from build123d import *

# Parameters (mm, degrees)
ESQUISSE1_W             = 330
ESQUISSE1_H             = 238
BOSS_EXTRU_1_DEPTH      = 6
ESQUISSE2_W             = 20
ESQUISSE2_H             = 6
ESQUISSE2_W_2           = 30
BOSS_EXTRU_2_DEPTH      = 6
ESQUISSE3_W             = 6
ESQUISSE3_H             = 10
ENL_V_MAT_EXTRU_1_DEPTH = 6
ESQUISSE4_R             = 1.4
ENL_V_MAT_EXTRU_2_DEPTH = 6


with BuildPart() as part:
    # Esquisse1 → Boss.-Extru.1 (new body)
    with BuildSketch(Plane.XY):
        Rectangle(ESQUISSE1_W, ESQUISSE1_H)
    extrude(amount=BOSS_EXTRU_1_DEPTH)

    # Esquisse2 → Boss.-Extru.2 (add)
    with BuildSketch(Plane.XY.offset(6)):
        with Locations((-125, 122)):
            Rectangle(ESQUISSE2_W, ESQUISSE2_H)
        with Locations((-50, 122)):
            Rectangle(ESQUISSE2_W_2, ESQUISSE2_H)
        with Locations((50, 122)):
            Rectangle(ESQUISSE2_W_2, ESQUISSE2_H)
        with Locations((125, 122)):
            Rectangle(ESQUISSE2_W, ESQUISSE2_H)
        with Locations((125, -122)):
            Rectangle(ESQUISSE2_W, ESQUISSE2_H)
        with Locations((50, -122)):
            Rectangle(ESQUISSE2_W_2, ESQUISSE2_H)
        with Locations((-50, -122)):
            Rectangle(ESQUISSE2_W_2, ESQUISSE2_H)
        with Locations((-125, -122)):
            Rectangle(ESQUISSE2_W, ESQUISSE2_H)
    extrude(amount=-BOSS_EXTRU_2_DEPTH)

    # Esquisse3 → Enlèv. mat.-Extru.1 (cut)
    with BuildSketch(Plane.XY.offset(6)):
        with Locations((-162, 84)):
            Rectangle(ESQUISSE3_W, ESQUISSE3_H)
        with Locations((-162, 34)):
            Rectangle(ESQUISSE3_W, ESQUISSE3_H)
        with Locations((-162, -34)):
            Rectangle(ESQUISSE3_W, ESQUISSE3_H)
        with Locations((-162, -84)):
            Rectangle(ESQUISSE3_W, ESQUISSE3_H)
        with Locations((162, -84)):
            Rectangle(ESQUISSE3_W, ESQUISSE3_H)
        with Locations((162, -34)):
            Rectangle(ESQUISSE3_W, ESQUISSE3_H)
        with Locations((162, 34)):
            Rectangle(ESQUISSE3_W, ESQUISSE3_H)
        with Locations((162, 84)):
            Rectangle(ESQUISSE3_W, ESQUISSE3_H)
    extrude(amount=-ENL_V_MAT_EXTRU_1_DEPTH, mode=Mode.SUBTRACT)

    # Esquisse4 → Enlèv. mat.-Extru.2 (cut)
    with BuildSketch(Plane.XY.offset(6)):
        with Locations((-125, 122)):
            Circle(ESQUISSE4_R)
        with Locations((-50, 122)):
            Circle(ESQUISSE4_R)
        with Locations((50, 122)):
            Circle(ESQUISSE4_R)
        with Locations((125, 122)):
            Circle(ESQUISSE4_R)
        with Locations((125, -122)):
            Circle(ESQUISSE4_R)
        with Locations((50, -122)):
            Circle(ESQUISSE4_R)
        with Locations((-50, -122)):
            Circle(ESQUISSE4_R)
        with Locations((-125, -122)):
            Circle(ESQUISSE4_R)
    extrude(amount=-ENL_V_MAT_EXTRU_2_DEPTH, mode=Mode.SUBTRACT)


solid = part.part
Input: part model. Units: mm. Frame: model coordinates. Coordinates: 2 decimals unless noted, no trailing zeros. Write each loop counter-clockwise with the first axis right and the second up, starting at its lowest first coordinate (ties: lowest second). Pieces come first, ordered by that corner, then holes. Notation, with made-up numbers: M 72,83 L 79,83 A15 cw 79,88 Z; hole C 66,34.5 d7. An arc over 180 degrees is marked long. Answer as a JSON object with one key per item and string values. Group by question number.
(1) Section A-A on z = 3.9. Give the number of separate pieces and of enclosed holes in the cut face, plus the area to 3 significant figures.
(2) Ray query, line 1 along Y through (x, z) = (50, 2.2); line 2 along Y through (x, z) = (6.5, 0.55); line 3 along X through (y, z) = (88, 2.7). Return the intervals inside material, ascending. Write a range as [from, to].
(3) Contact query for flat-ended pins moving along their axis: P1, Ø3, axis at y = 32.5, z = 2.5, coming from the +X side; P2, Ø3, axis at x = 125, y = -122, coming from the +Z side; P3, Ø2.5, axis at x = 50, y = 122, coming from the +Z side; P4, Ø3, axis at y = -123.5, z = 3, coming from the +X side. Output: stop coordinate, or through.
(4) Section B-B on x = -141. Output: boundary loops of the cut face in (y, z).
Result set:
{
 "1": {"separate pieces": "1", "enclosed holes": "8", "area": "79,200 mm2"},
 "2": {"line 1": "y = [-125, -123.4], [-120.6, 120.6], [123.4, 125]", "line 2": "y = [-119, 119]", "line 3": "x = [-159, 159]"},
 "3": {"P1": "stops at x = 159", "P2": "stops at z = 6", "P3": "passes through", "P4": "stops at x = 135"},
 "4": {"outline": "M -119,0 L 119,0 L 119,6 L -119,6 Z"}
}
